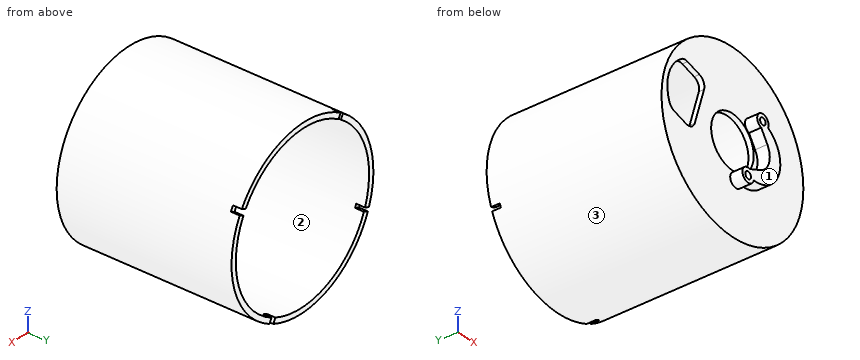
```python
from build123d import *

# Parameters (mm, degrees)
SKETCH1_R           = 50
BOSS_EXTRUDE1_DEPTH = 100
SHELL1_T            = -3
CUT_EXTRUDE1_REACH  = 124.474
SKETCH2_R           = 15
BOSS_EXTRUDE2_DEPTH = 7
SKETCH4_R           = 2
CUT_EXTRUDE2_DEPTH  = 4
CUT_EXTRUDE3_DEPTH  = 3
FILLET1_R           = 5
CAVITY1_START       = 94.95
CAVITY1_DEPTH       = 5.05


# Read off the part's stored shape, not the designer's step: Cavity1
with BuildPart() as part:
    # Sketch1 → Boss-Extrude1 (new body)
    with BuildSketch(Plane(origin=(0, 0, 0), x_dir=(1, 0, 0), z_dir=(0, 1, 0))):
        with Locations(Location((0, 0, 0), (0, 0, 270))):
            Circle(SKETCH1_R)
    extrude(amount=BOSS_EXTRUDE1_DEPTH)

    # Shell1
    shell1_openings = [part.faces().sort_by_distance(p)[0] for p in [
        (0, 100, 0),
    ]]
    offset(amount=SHELL1_T, openings=shell1_openings, kind=Kind.INTERSECTION)

    # Sketch2 → Cut-Extrude1 (cut, up to next)
    with BuildSketch(Plane.XZ, mode=Mode.PRIVATE) as cut_extrude1_sk1:
        with Locations(Location((0, 0, 0), (0, 0, 270))):
            Circle(SKETCH2_R)
    cut_extrude1_tool1 = extrude(cut_extrude1_sk1.sketch, amount=-CUT_EXTRUDE1_REACH, mode=Mode.PRIVATE) & part.part
    add(cut_extrude1_tool1.solids().sort_by_distance((0, 0, 0))[0], mode=Mode.SUBTRACT)

    # Sketch3 → Boss-Extrude2 (add)
    with BuildSketch(Plane.XZ):
        with BuildLine():
            Line((11.656771923, 10.505696947), (15.97605159, 3.771914714))
            ThreePointArc((15.97605159, 3.771914714), (17.208044811, -5.36712002), (10.999048015, -12.185339871))
            Line((10.999048015, -12.185339871), (3.617532023, -15.269690962))
            ThreePointArc((3.617532023, -15.269690962), (-1.003618951, -21.145948661), (6.356204016, -19.835053254))
            ThreePointArc((6.356204016, -19.835053254), (24.343421913, -7.592615462), (16.505212694, 12.704669259))
            ThreePointArc((16.505212694, 12.704669259), (11.195588228, 17.967114404), (11.656771923, 10.505696947))
        make_face()
    extrude(amount=BOSS_EXTRUDE2_DEPTH)

    # Sketch4 → Cut-Extrude2 (cut)
    with BuildSketch(Plane.XZ.offset(7)):
        with Locations(Location((12.847770427, 14.324272933, 0), (0, 0, 270))):
            Circle(SKETCH4_R)
        with Locations(Location((2.426533519, -19.088266948, 0), (0, 0, 270))):
            Circle(SKETCH4_R)
    extrude(amount=-CUT_EXTRUDE2_DEPTH, mode=Mode.SUBTRACT)

    # Sketch5 → Cut-Extrude3 (cut)
    with BuildSketch(Plane.XZ):
        with BuildLine():
            Line((-28.03113406, -8.017376473), (-18.503146029, 22.531231418))
            Line((-18.503146029, 22.531231418), (-33.777449975, 27.295225433))
            ThreePointArc((-33.777449975, 27.295225433), (-44.86826784, 13.99423242), (-43.305438005, -3.253382458))
            Line((-43.305438005, -3.253382458), (-28.03113406, -8.017376473))
        make_face()
    extrude(amount=-CUT_EXTRUDE3_DEPTH, mode=Mode.SUBTRACT)

    # Fillet1
    fillet1_edges = [part.edges().sort_by_distance(p)[0] for p in [
        (-33.777449975, 1.5, 27.295225433),
        (-18.503146029, 1.5, 22.531231418),
        (-28.03113406, 1.5, -8.017376473),
        (-43.305438005, 1.5, -3.253382458),
    ]]
    fillet(fillet1_edges, radius=FILLET1_R)

    # Cavity1 outline → Cavity1 (cut)
    with BuildSketch(Plane(origin=(0, 0, 0), x_dir=(1, 0, 0), z_dir=(0, 1, 0)).offset(CAVITY1_START)):
        with BuildLine():
            ThreePointArc((19.102530443, 42.942907804), (20.477537397, 42.30449695), (21.831239809, 41.622073091))
            Line((21.831239809, 41.622073091), (23.224723201, 44.278801161))
            ThreePointArc((23.224723201, 44.278801161), (21.871785206, 44.962484495), (20.498743854, 45.604840756))
            Line((20.498743854, 45.604840756), (19.102530443, 42.942907804))
        make_face()
        with BuildLine():
            Line((44.278801161, -23.224723201), (41.622073091, -21.831239809))
            ThreePointArc((41.622073091, -21.831239809), (40.896346213, -23.162229305), (40.128071352, -24.469121144))
            Line((40.128071352, -24.469121144), (42.790004304, -25.865334555))
            ThreePointArc((42.790004304, -25.865334555), (43.55441916, -24.556314293), (44.278801161, -23.224723201))
        make_face()
        with BuildLine():
            ThreePointArc((-44.105134018, 16.239986245), (-43.745876837, 17.184244522), (-43.366406458, 18.120562655))
            Line((-43.366406458, 18.120562655), (-46.134474955, 19.277194314))
            ThreePointArc((-46.134474955, 19.277194314), (-46.514536622, 18.341152714), (-46.875608808, 17.397623369))
            Line((-46.875608808, 17.397623369), (-44.105134018, 16.239986245))
        make_face()
        with BuildLine():
            Line((-26.99549792, -42.086138954), (-25.375768045, -39.560970617))
            ThreePointArc((-25.375768045, -39.560970617), (-26.220241948, -39.006395786), (-27.052600539, -38.43379768))
            Line((-27.052600539, -38.43379768), (-28.673738451, -40.961161156))
            ThreePointArc((-28.673738451, -40.961161156), (-27.840301063, -41.532127765), (-26.99549792, -42.086138954))
        make_face()
    extrude(amount=CAVITY1_DEPTH, mode=Mode.SUBTRACT)


solid = part.part
```
Geometry check sheet. Reference: the model listing, model coordinates, mm. Face numbers are marked on the shaded views. Give positions to 0.01 mm unless a question says otherwise; leave off trailing zeros. Write each loop counter-clockwise with the first axis right and the second up, starting at its lowest first coordinate (ties: lowest second). Pieces come first, ordered by that corner, then holes.
1) Section check B-B, the plane x = -7. Record the boundary of the cut face in (y, z), and give its area (3 significant figures).
2) Release check for a two-part mould opening along Z. For the marked faces 1, 2 and 3 record: pulls with the +Z half, pulls with the -Z half, needs draft (parallel to the pull), parting line crosses it, or undercut.
3) Gauge pin test, flat ends, axial feed: pin 1 (2 mm diameter, centred on x = -27, y = 48, fed in from -Z); pin 2 (6 mm diameter, centred on y = 49, z = -10.5, fed in from -X); pin 3 (4.5 mm diameter, centred on x = 3, z = -19, fed in from -Y); pin 4 (8 mm diameter, centred on x = -4.5, y = 83, fed in from -Z). Record the tip position at first contact, or that the pin passes through.
4) Section check A-A, the plane z = 7.5. Record the boundary of the cut face in (x, y).
5) Section check C-C, the plane z = -31. Record the boundary of the cut face in (x, y).
6) Material ranges on L1, parallel to X at y = 31.5, z = -0.5; L2, parallel to X at y = 1.45, z = 0, recorded low to high.
7) Section check D-D, the plane y = 40. Record the boundary of the cut face in (x, z), and give its area (3 significant figures).
Computed:
1. outline: (0, -49.51) - (100, -49.51) - (100, -46.48) - (3, -46.48) - (3, -13.27) - (0, -13.27) - close; (0, 13.27) - (3, 13.27) - (3, 46.48) - (100, 46.48) - (100, 49.51) - (0, 49.51) - close
1. area: 806 mm2
2. face 1: needs draft
2. face 2: undercut
2. face 3: parting line crosses it
3. pin 1: stops at z = -42.71
3. pin 2: stops at x = -49.43
3. pin 3: stops at y = -7
3. pin 4: stops at z = -50
4. outline: (-49.43, 0) - (-45.89, 0) - (-45.89, 3) - (-46.4, 3) - (-46.4, 100) - (-49.43, 100) - close; (-23.19, 0) - (-12.99, 0) - (-12.99, 3) - (-23.19, 3) - close; (12.99, 0) - (13.58, 0) - (13.58, -7) - (22.08, -7) - (22.08, 0) - (49.43, 0) - (49.43, 100) - (46.4, 100) - (46.4, 3) - (12.99, 3) - close
5. outline: (-39.23, 0) - (39.23, 0) - (39.23, 100) - (35.33, 100) - (35.33, 3) - (-35.33, 3) - (-35.33, 100) - (-39.23, 100) - close
6. L1: x = -50 to -47, 47 to 50
6. L2: x = -50 to -44.7, -25.53 to -15, 15 to 50
7. outline: circle Ø100 at (0, 0); hole circle Ø94 at (0, 0)
7. area: 914 mm2
